Work out the finished part from the listing and answer in its coordinate system (mm). Round coordinates to 2 decimals unless told otherwise and drop trailing zeros. Order: outer loops, then holes, each group sorted by start corner. A loop starts at its lowest first (then second) coordinate and runs counter-clockwise, first axis right, second up. Notation, with made-up numbers: (27.5, 26.5) -> (36.5, 26.5) arc R16 cw to (36.5, 49.5) -> close; hole circle Ø2 at (86.25, 42.25). An arc over 180 degrees is marked (long way). Use one line per item in the form item = value.
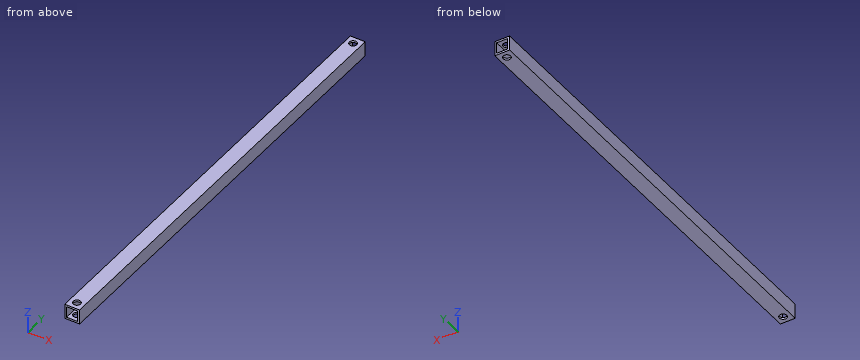
Autodesk Inventor part; units mm, degrees
ref_plane "YZ Plane" through (0, 0, 0) normal (1, 0, 0) x (0, 1, 0)
ref_plane "XZ Plane" through (0, 0, 0) normal (0, 1, 0) x (-1, 0, 0)
ref_plane "XY Plane" through (0, 0, 0) normal (0, 0, 1) x (1, 0, 0)
sketch "Sketch1" plane through (0, 0, 0) normal (0, 1, 0) x (-1, 0, 0)
  line L0 (0, 0) -> (25.4, 0)
  line L1 (25.4, 0) -> (25.4, -25.4)
  line L2 (25.4, -25.4) -> (0, -25.4)
  line L3 (0, -25.4) -> (0, 0)
  line L4 (22.225, -3.175) -> (3.175, -3.175)
  line L5 (3.175, -3.175) -> (3.175, -22.225)
  line L6 (3.175, -22.225) -> (22.225, -22.225)
  line L7 (22.225, -22.225) -> (22.225, -3.175)
  dimension "d0" = 25.4
  dimension "d1" = 25.4
  dimension "d2" = 3.175
extrude "Extrusion1" add sketch "Sketch1" along normal blind 762
sketch "Sketch2" plane through (0, 0, -25.4) normal (0, 0, -1) x (-1, 0, 0)
  circle A0 centre (12.7, 12.7) radius 6.35
  circle A1 centre (12.7, 749.3) radius 6.35
  line L0 (25.4, 0) -> (25.4, 762)
  line L1 (22.225, 762) -> (3.175, 762)
  line L2 (25.4, 0) -> (0, 0)
  dimension "d5" = 12.7
  dimension "d6" = 12.7
  dimension "d7" = 12.7
  dimension "d8" = 12.7
  dimension "d9" = 12.7
  dimension "d10" = 12.7
extrude "Extrusion2" cut sketch "Sketch2" against normal blind 25.4
properties part number "upper arm"
Item 1: Consider line 1 along Y through (x, z) = (-12.7, -1.2); line 2 along X through (y, z) = (604, -6.5) (3 decimals). Determine where each line is inside the solid, lowest interval first.
Findings:
line_1 = 0 to 6.35, 19.05 to 742.95, 755.65 to 762
line_2 = -25.4 to -22.225, -3.175 to 0
Item 2: A flat-ended cylindrical pin translates along its axis: P1, Ø3, axis at x = -4.5, z = -13, coming from the -Y side. Find the tip coordinate at first contact, or state that the pin passes through.
Findings:
P1 = 0
Item 3: The part is cut by section A-A, the plane x = -12.7. Give the vertices of the cut face in (y, z) (3 decimals), and give its area (3 significant figures).
Findings:
outline = (0, -25.4) -> (6.35, -25.4) -> (6.35, -22.225) -> (0, -22.225) -> close; (0, -3.175) -> (6.35, -3.175) -> (6.35, 0) -> (0, 0) -> close; (19.05, -25.4) -> (742.95, -25.4) -> (742.95, -22.225) -> (19.05, -22.225) -> close; (19.05, -3.175) -> (742.95, -3.175) -> (742.95, 0) -> (19.05, 0) -> close; (755.65, -25.4) -> (762, -25.4) -> (762, -22.225) -> (755.65, -22.225) -> close; (755.65, -3.175) -> (762, -3.175) -> (762, 0) -> (755.65, 0) -> close
area = 4,680 mm^2
Item 4: The part is cut by section D-D, the plane y = 259. Give the vertices of the cut face in (x, z) (3 decimals).
Findings:
outline = (-25.4, -25.4) -> (0, -25.4) -> (0, 0) -> (-25.4, 0) -> close; hole (-22.225, -22.225) -> (-3.175, -22.225) -> (-3.175, -3.175) -> (-22.225, -3.175) -> close
Item 5: The part is cut by section B-B, the plane z = -13.25. Give the vertices of the cut face in (x, y) (3 decimals).
Findings:
outline = (-25.4, 0) -> (-22.225, 0) -> (-22.225, 762) -> (-25.4, 762) -> close; (-3.175, 0) -> (0, 0) -> (0, 762) -> (-3.175, 762) -> close
Item 6: The part is cut by section C-C, the plane y = 12.7. Give the vertices of the cut face in (x, z) (3 decimals).
Findings:
outline = (-25.4, -25.4) -> (-19.05, -25.4) -> (-19.05, -22.225) -> (-22.225, -22.225) -> (-22.225, -3.175) -> (-19.05, -3.175) -> (-19.05, 0) -> (-25.4, 0) -> close; (-6.35, -25.4) -> (0, -25.4) -> (0, 0) -> (-6.35, 0) -> (-6.35, -3.175) -> (-3.175, -3.175) -> (-3.175, -22.225) -> (-6.35, -22.225) -> close
